Geometry: final body of the model. Coordinates: model frame, mm. A direction names the side the tool comes from. Give positions to 0.01 mm unless a question says otherwise; leave off trailing zeros. Write each loop counter-clockwise with the first axis right and the second up, starting at its lowest first coordinate (ties: lowest second). Pieces come first, ordered by that corner, then holes.
Q1. Section A-A (x = 0). Return the cut outline in (y, z).
Q2. Pin query (flat end, axial travel): pin 1 Ø1 at (x, y) = (-1.5, -15) entering from +Z. Return the tip coordinate at first contact, or that it passes through.
Q3. Section B-B (y = 0). Return the cut outline in (x, z), plus the area to 3 significant figures.
Q4. Mould query, pull axis Y, two halves, no side actions, for faces 3 (the cylindrical face through (-20.45, 20.1, 1.77)), 4 (the cylindrical face through (-17.032, 15.128, 1.775)), 5 (the flat face through (0, 19, 3.5)). Classes: +Y half, -Y half, draft (parallel to the pull), parting line (faces both ways), or undercut.
Q5. Section C-C (z = 2.45). Return the cut outline in (x, y), plus the area to 3 significant figures.
Q6. Reachability of faces 1 (the cylindrical face through (-18.684, -16.563, 1.775)), 2 (the flat face through (-8, 12, 1.75)) from +Z, -Z, +X, -X, +Y, -Y: full face, straight path, thin tool, end or side. Return the list, or none.
Q7. Line query: line 1 (X direction, y = 0, z = 1.65); line 2 (Y direction, x = 0, z = 0.7); line 3 (X direction, y = -18, z = 2.5). Output: solid intervals per line, ascending.
Q8. Section D-D (y = 16). Return the cut outline in (x, z).
from build123d import *

# Parameters (mm, degrees)
SKETCH1_W            = 42.614634146
SKETCH1_H            = 42
SKETCH1_R            = 14
BOSS_EXTRUDE1_DEPTH  = 3.5
SKETCH2_R            = 17.5
CUT_EXTRUDE1_DEPTH   = 1.75
M3_CLEARANCE_HOLE1_D = 3.6
FILLET1_R            = 3


with BuildPart() as part:
    # Sketch1 → Boss-Extrude1 (new body)
    with BuildSketch(Plane.XY):
        Rectangle(SKETCH1_W, SKETCH1_H)
        Circle(SKETCH1_R, mode=Mode.SUBTRACT)
    extrude(amount=BOSS_EXTRUDE1_DEPTH)

    # Sketch2 → Cut-Extrude1 (cut)
    with BuildSketch(Plane.XY.offset(3.5)):
        Circle(SKETCH2_R)
    extrude(amount=-CUT_EXTRUDE1_DEPTH, mode=Mode.SUBTRACT)

    # M3 Clearance Hole1 (through all)
    with Locations(Plane(origin=(0, 0, 0), x_dir=(-1, 0, 0), z_dir=(0, 0, -1))):
        with Locations((-16.642079068, -16.885621688), (-16.885621688, 16.642079068), (16.642079068, 16.885621688), (16.885621688, -16.642079068)):
            Hole(M3_CLEARANCE_HOLE1_D / 2)

    # Fillet1
    fillet1_edges = [part.edges().sort_by_distance(p)[0] for p in [
        (-21.307317073, 21, 1.75),
        (21.307317073, 21, 1.75),
        (21.307317073, -21, 1.75),
        (-21.307317073, -21, 1.75),
    ]]
    fillet(fillet1_edges, radius=FILLET1_R)


solid = part.part
Computed:
1. outline: (-21, 0) - (-14, 0) - (-14, 1.75) - (-17.5, 1.75) - (-17.5, 3.5) - (-21, 3.5) - close; (14, 0) - (21, 0) - (21, 3.5) - (17.5, 3.5) - (17.5, 1.75) - (14, 1.75) - close
2. pin 1: stops at z = 1.75
3. outline: (-21.31, 0) - (-14, 0) - (-14, 1.75) - (-17.5, 1.75) - (-17.5, 3.5) - (-21.31, 3.5) - close; (14, 0) - (21.31, 0) - (21.31, 3.5) - (17.5, 3.5) - (17.5, 1.75) - (14, 1.75) - close
3. area: 38.9 mm2
4. face 3: +Y half
4. face 4: undercut
4. face 5: draft
5. outline: (-21.31, -18) arc R3 ccw to (-18.31, -21) - (18.31, -21) arc R3 ccw to (21.31, -18) - (21.31, 18) arc R3 ccw to (18.31, 21) - (-18.31, 21) arc R3 ccw to (-21.31, 18) - close; hole circle Ø3.6 at (-16.89, -16.64); hole circle Ø3.6 at (-16.64, 16.89); hole circle Ø35 at (0, 0); hole circle Ø3.6 at (16.64, -16.89); hole circle Ø3.6 at (16.89, 16.64)
5. area: 779 mm2
6. face 1: +Z, -Z
6. face 2: +Z
7. line 1: x = -21.31 to -14, 14 to 21.31
7. line 2: y = -21 to -14, 14 to 21
7. line 3: x = -21.31 to -18.07, -15.7 to 15.23, 18.06 to 21.31
8. outline: (-21.31, 0) - (-18.21, 0) - (-18.21, 3.5) - (-21.31, 3.5) - close; (-15.08, 0) - (15.2, 0) - (15.2, 3.5) - (7.09, 3.5) - (7.09, 1.75) - (-7.09, 1.75) - (-7.09, 3.5) - (-15.08, 3.5) - close; (18.57, 0) - (21.31, 0) - (21.31, 3.5) - (18.57, 3.5) - close
